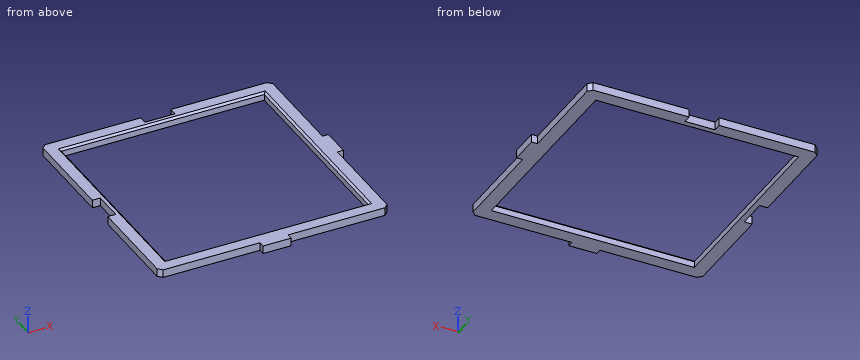
```python
from build123d import *

# Parameters (mm, degrees)
F0_W     = 101.5
F0_H     = 101.5
F1_DEPTH = 4
F2_SIZE  = 2
F3_SIZE  = 1


with BuildPart() as f1:
    # F0 (on Top) → F1 (new body)
    with BuildSketch(Plane.XY):
        Polygon((-7.5, 57.5), (-57.5, 57.5), (-57.5, 7.5), (-53.5, 7.5), (-53.5, -7.5), (-57.5, -7.5), (-57.5, -57.5), (-7, -57.5), (-7, -60.5), (7, -60.5), (7, -57.5), (57.5, -57.5), (57.5, -7.25), (60.5, -7.25), (60.5, 7.25), (57.5, 7.25), (57.5, 57.5), (7.5, 57.5), (7.5, 53.5), (-7.5, 53.5), align=None)
        Rectangle(F0_W, F0_H, mode=Mode.SUBTRACT)
    extrude(amount=F1_DEPTH)

    # F2
    f2_edges = [f1.edges().sort_by_distance(p)[0] for p in [
        (-57.5, -57.5, 2),
        (57.5, -57.5, 2),
        (57.5, 57.5, 2),
        (-57.5, 57.5, 2),
    ]]
    chamfer(f2_edges, length=F2_SIZE)

    # F3
    f3_edges = [f1.edges().sort_by_distance(p)[0] for p in [
        (-50.75, 0, 4),
        (0, 50.75, 4),
        (50.75, 0, 4),
        (0, -50.75, 4),
    ]]
    chamfer(f3_edges, length=F3_SIZE)


solid = f1.part
```
CAD build for the part. Positions are in the model's coordinates, mm. Round coordinates to 2 decimals unless told otherwise and drop trailing zeros. Loops run counter-clockwise (first coordinate to the right, second up) from the corner with the lowest first, then second, coordinate; pieces in that order, holes last. Notation, with made-up numbers: M 62.5,21.5 L 74.5,21.5 A32 cw 74.5,59.5 Z; hole C 72,-36 d7. An arc over 180 degrees is marked long. Use a Markdown table: item, result. Add a question column.
(1) Drill centre lines: line 1 (Y direction, x = -36, z = 1.3); line 2 (X direction, y = 5, z = 1.5). Where is each one in solid material? Low to high.
(2) Cut at A-A (y = -19.5). Give the cut face in (x, z).
(3) Flat gauge pins, fed straight in: pin 1 (1.2 mm diameter, centred on y = 55.5, z = 2.5, fed in from +X); pin 2 (0.9 mm diameter, centred on x = 59, z = 1, fed in from -Y); pin 3 (2 mm diameter, centred on y = -3, z = 1.5, fed in from -X). Where does each tip first touch, or does it go through?
(4) Cut at C-C (z = 2). Give the cut face in (x, y).
Geometry says:
| question | item | result |
|---|---|---|
| 1 | line 1 | y = -57.5 to -50.75, 50.75 to 57.5 |
| 1 | line 2 | x = -53.5 to -50.75, 50.75 to 60.5 |
| 2 | outline | M -57.5,0 L -50.75,0 L -50.75,3 L -51.75,4 L -57.5,4 Z; M 50.75,0 L 57.5,0 L 57.5,4 L 51.75,4 L 50.75,3 Z |
| 3 | pin 1 | stops at x = 57.5 |
| 3 | pin 2 | stops at y = -7.25 |
| 3 | pin 3 | stops at x = -53.5 |
| 4 | outline | M -57.5,-55.5 L -55.5,-57.5 L -7,-57.5 L -7,-60.5 L 7,-60.5 L 7,-57.5 L 55.5,-57.5 L 57.5,-55.5 L 57.5,-7.25 L 60.5,-7.25 L 60.5,7.25 L 57.5,7.25 L 57.5,55.5 L 55.5,57.5 L 7.5,57.5 L 7.5,53.5 L -7.5,53.5 L -7.5,57.5 L -55.5,57.5 L -57.5,55.5 L -57.5,7.5 L -53.5,7.5 L -53.5,-7.5 L -57.5,-7.5 Z; hole M -50.75,-50.75 L 50.75,-50.75 L 50.75,50.75 L -50.75,50.75 Z |
